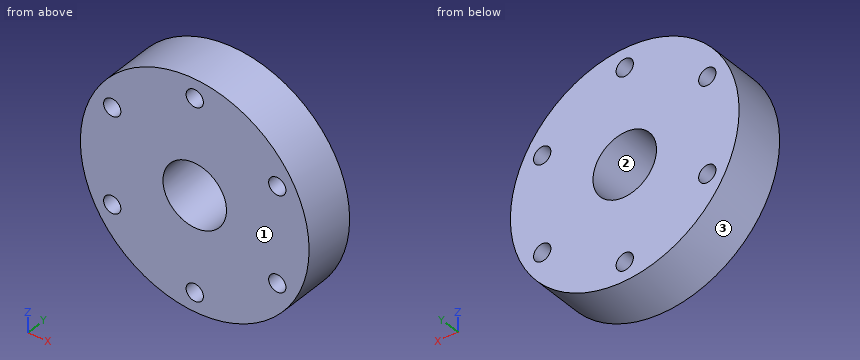
Autodesk Inventor part; units mm, degrees
ref_plane "YZ Plane" through (0, 0, 0) normal (1, 0, 0) x (0, 1, 0)
ref_plane "XZ Plane" through (0, 0, 0) normal (0, 1, 0) x (-1, 0, 0)
ref_plane "XY Plane" through (0, 0, 0) normal (0, 0, 1) x (1, 0, 0)
sketch "Sketch1" plane through (0, 0, 0) normal (0, 1, 0) x (-1, 0, 0)
  circle A0 centre (0, 0) radius 23.8125 construction
  circle A1 centre (0, 23.8125) radius 2.159
  line L0 (0, 0) -> (0, 23.8125) construction
  line L1 (0, 23.8125) -> (20.6222, 11.9062) construction
  line L2 (20.6222, 11.9062) -> (20.6222, -11.9062) construction
  line L3 (20.6222, -11.9062) -> (0, -23.8125) construction
  line L4 (0, -23.8125) -> (-20.6222, -11.9063) construction
  line L5 (-20.6222, -11.9063) -> (-20.6222, 11.9062) construction
  line L6 (-20.6222, 11.9062) -> (0, 23.8125) construction
  circle A2 centre (-20.6222, 11.9062) radius 2.159
  circle A3 centre (-20.6222, -11.9063) radius 2.159
  circle A4 centre (0, -23.8125) radius 2.159
  circle A5 centre (20.6222, -11.9062) radius 2.159
  circle A6 centre (20.6222, 11.9062) radius 2.159
  circle A7 centre (0, 0) radius 28.575
  circle A8 centre (0, 0) radius 7.9375
  dimension "d0" = 47.625
  dimension "d1" = 4.318
  dimension "d2" = 4.318
  dimension "d3" = 4.318
  dimension "d4" = 4.318
  dimension "d5" = 4.318
  dimension "d6" = 4.318
  dimension "d7" = 57.15
  dimension "d10" = 15.875
extrude "Extrusion2" add sketch "Sketch1" along normal blind 12.7762
properties part number "spacer" material "Aluminum 6061"
Geometry: final body of the model. Coordinates: model frame, mm. Face numbers are marked on the shaded views. Round coordinates to 2 decimals unless told otherwise and drop trailing zeros. Write each loop counter-clockwise with the first axis right and the second up, starting at its lowest first coordinate (ties: lowest second). Pieces come first, ordered by that corner, then holes. Notation, with made-up numbers: (70.5, 29) -> (98.5, 29) arc R13 ccw to (98.5, 48) -> close; hole circle Ø4 at (24, 10). An arc over 180 degrees is marked (long way). Return JSON: item names as keys, results as strings.
Q1. Section D-D on x = -20. Return the cut outline in (y, z).
From the geometry:
{"outline": "(0, -20.41) -> (12.78, -20.41) -> (12.78, -13.97) -> (0, -13.97) -> close; (0, -9.84) -> (12.78, -9.84) -> (12.78, 9.84) -> (0, 9.84) -> close; (0, 13.97) -> (12.78, 13.97) -> (12.78, 20.41) -> (0, 20.41) -> close"}
Q2. Mould query, pull axis Z, two halves, no side actions, for the marked faces 1, 2 and 3. Classes: +Z half, -Z half, draft (parallel to the pull), parting line (faces both ways), or undercut.
From the geometry:
{"face 1": "draft", "face 2": "undercut", "face 3": "parting line"}
Q3. Section B-B on z = 0. Return the cut outline in (x, y) (1 decimal).
From the geometry:
{"outline": "(-28.6, 0) -> (-7.9, 0) -> (-7.9, 12.8) -> (-28.6, 12.8) -> close; (7.9, 0) -> (28.6, 0) -> (28.6, 12.8) -> (7.9, 12.8) -> close"}
Q4. Section A-A on x = 0. Return the cut outline in (y, z) (1 decimal).
From the geometry:
{"outline": "(0, -28.6) -> (12.8, -28.6) -> (12.8, -26) -> (0, -26) -> close; (0, -21.7) -> (12.8, -21.7) -> (12.8, -7.9) -> (0, -7.9) -> close; (0, 7.9) -> (12.8, 7.9) -> (12.8, 21.7) -> (0, 21.7) -> close; (0, 26) -> (12.8, 26) -> (12.8, 28.6) -> (0, 28.6) -> close"}
Q5. First-contact query: pin 1 Ø3 at (y, z) = (6, 2.5) entering from +X; pin 2 Ø5 at (x, y) = (15.5, 6) entering from -Z; pin 3 Ø5 at (x, z) = (-20.62, -11.91) entering from -Y; pin 4 Ø3 at (y, z) = (7.5, 7) entering from -X. Flat tips, straight axial feed; report the tip coordinate or a pass-through.
From the geometry:
{"pin 1": "x = 28.56", "pin 2": "z = -25.45", "pin 3": "y = 0", "pin 4": "x = -28.04"}
Q6. Section C-C on y = 4.5. Give the number of separate pieces and of enclosed holes in the cut face, and give its area (3 significant figures).
From the geometry:
{"separate pieces": "1", "enclosed holes": "7", "area": "2,280 mm2"}
Q7. Ray query, line 1 (Z direction, x = 0, y = 9) (1 decimal); line 2 (Z direction, x = -21.5, y = 10); line 3 (Z direction, x = -0.5, y = 6.25). Return the intervals inside material, ascending.
From the geometry:
{"line 1": "-28.6 to -26, -21.7 to -7.9, 7.9 to 21.7, 26 to 28.6", "line 2": "-18.82 to -13.88, -9.93 to 9.93, 13.88 to 18.82", "line 3": "-28.57 to -25.91, -21.71 to -7.92, 7.92 to 21.71, 25.91 to 28.57"}
